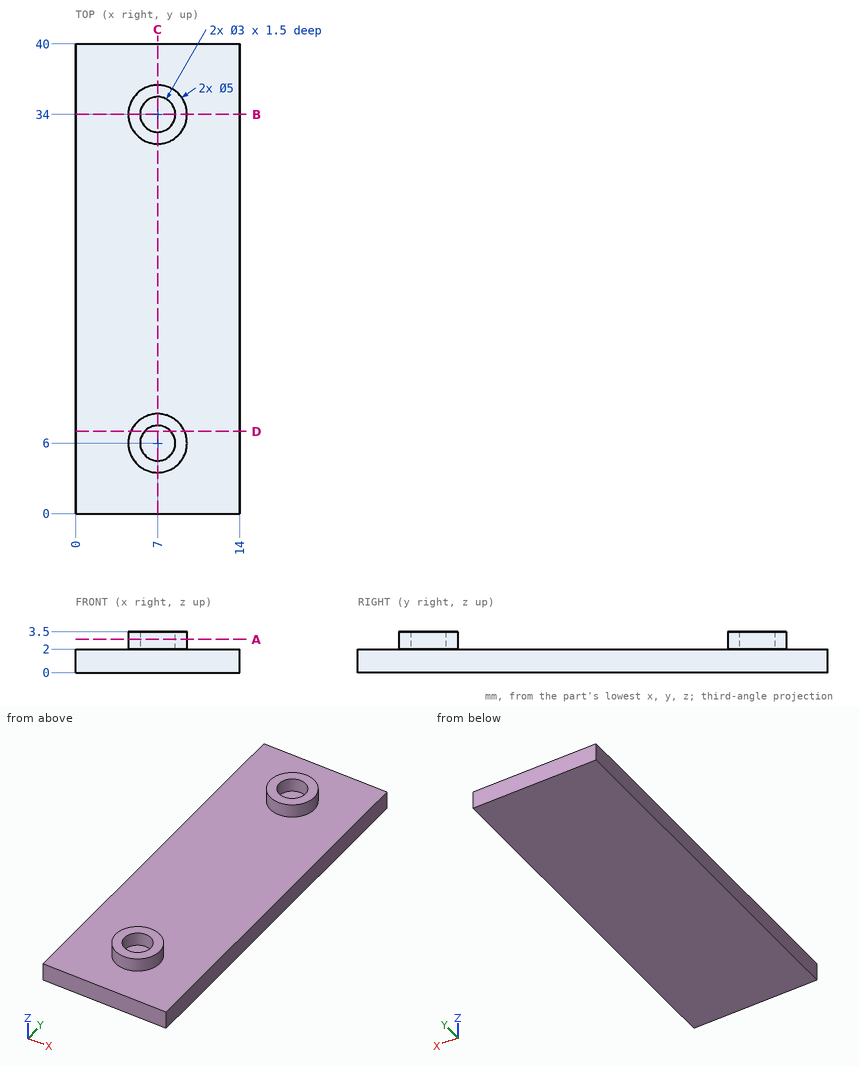
Check sheet for the drawn part. Datum: minimum x, y, z corner. Units: mm. Round coordinates to 2 decimals unless told otherwise and drop trailing zeros. Order: outer loops, then holes, each group sorted by start corner. A loop starts at its lowest first (then second) coordinate and runs counter-clockwise, first axis right, second up.
1) Go/stop test with flat-tipped pins: pin 1 Ø4 at (x, y) = (9, 21.5) entering from +Z; pin 2 Ø3.5 at (x, y) = (7, 6.5) entering from +Z. Record where each tip stops, or that it passes through.
2) Section check D-D (y = 7). Record the boundary of the cut face in (x, z).
3) Section check C-C (x = 7). Record the boundary of the cut face in (y, z).
4) Section check B-B (y = 34). Record the boundary of the cut face in (x, z), and give its area (3 significant figures).
5) Section check A-A (z = 2.85). Record the boundary of the cut face in (x, y), and give its area (3 significant figures).
6) Scan lines: line 1 (Y direction, x = 7, z = 2.75); line 2 (Z direction, x = 13.25, y = 14.5); line 3 (X direction, y = 36, z = 2.7). Record each from-to range of solid material in increasing order.
Result:
1. pin 1: stops at z = 2
1. pin 2: stops at z = 3.5
2. outline: (0, 0) - (14, 0) - (14, 2) - (9.29, 2) - (9.29, 3.5) - (8.12, 3.5) - (8.12, 2) - (5.88, 2) - (5.88, 3.5) - (4.71, 3.5) - (4.71, 2) - (0, 2) - close
3. outline: (0, 0) - (40, 0) - (40, 2) - (36.5, 2) - (36.5, 3.5) - (35.5, 3.5) - (35.5, 2) - (32.5, 2) - (32.5, 3.5) - (31.5, 3.5) - (31.5, 2) - (8.5, 2) - (8.5, 3.5) - (7.5, 3.5) - (7.5, 2) - (4.5, 2) - (4.5, 3.5) - (3.5, 3.5) - (3.5, 2) - (0, 2) - close
4. outline: (0, 0) - (14, 0) - (14, 2) - (9.5, 2) - (9.5, 3.5) - (8.5, 3.5) - (8.5, 2) - (5.5, 2) - (5.5, 3.5) - (4.5, 3.5) - (4.5, 2) - (0, 2) - close
4. area: 31.0 mm2
5. outline: circle Ø5 at (7, 6); circle Ø5 at (7, 34); hole circle Ø3 at (7, 6); hole circle Ø3 at (7, 34)
5. area: 25.1 mm2
6. line 1: y = 3.5 to 4.5, 7.5 to 8.5, 31.5 to 32.5, 35.5 to 36.5
6. line 2: z = 0 to 2
6. line 3: x = 5.5 to 8.5
